Could you check a few things on this drawing? It's one solid part, dimensions in mm from its lowest x, y, z. A direction names the side the tool comes from. Coordinates: 2 decimals unless noted, no trailing zeros. Loops run counter-clockwise (first coordinate to the right, second up) from the corner with the lowest first, then second, coordinate; pieces in that order, holes last. Notation, with made-up numbers: (40, 77.5) -> (52, 77.5) arc R12 cw to (52, 98.5) -> close; hole circle Ø10 at (88, -15.5). An arc over 180 degrees is marked (long way). One line per question, with ' | ' between items. Start each with the question number.
(1) If we mould it in two halves opening along Z, with no side actions, what happens to the marked faces 1, 2 and 3? For each: pulls with the +Z half, pulls with the -Z half, needs draft (parallel to the pull), parting line crosses it, or undercut.
(2) I'm going to push flat-ended pins straight in: pin 1 Ø3 at (x, y) = (2.5, 4) entering from -Z; pin 2 Ø3 at (x, z) = (7.5, 1.5) entering from +Y; pin 3 Ø4 at (x, y) = (7, 6) entering from -Z; pin 4 Ø1 at (x, y) = (3.5, 3.5) entering from +Z. Where does each tip first touch, or does it pass through?
(3) Suppose I cut it at C-C (y = 1). Please give me the cut outline in (x, z), plus the area to 3 significant figures.
(4) Suppose I cut it at A-A (z = 7.5). Please give me the cut outline in (x, y) (1 decimal).
(5) Suppose I cut it at B-B (x = 6.25). Please give me the cut outline in (y, z) (1 decimal).
(6) Which directions (+Z, -Z, +X, -X, +Y, -Y) give clear straight access to the entire face, cutting with the end or side of a thin tool? Please do the marked faces 4 and 5.
(7) Suppose I cut it at D-D (x = 3.25). Please give me the cut outline in (y, z) (1 decimal), plus the area to 3 significant figures.
(8) If I drill on line 1 along Z through (x, y) = (5.5, 3.25) (1 decimal); line 2 along Y through (x, z) = (10.75, 6); line 3 along X through (y, z) = (5.5, 7.25) (1 decimal), over which ranges is the centre line in solid material (lowest first)?
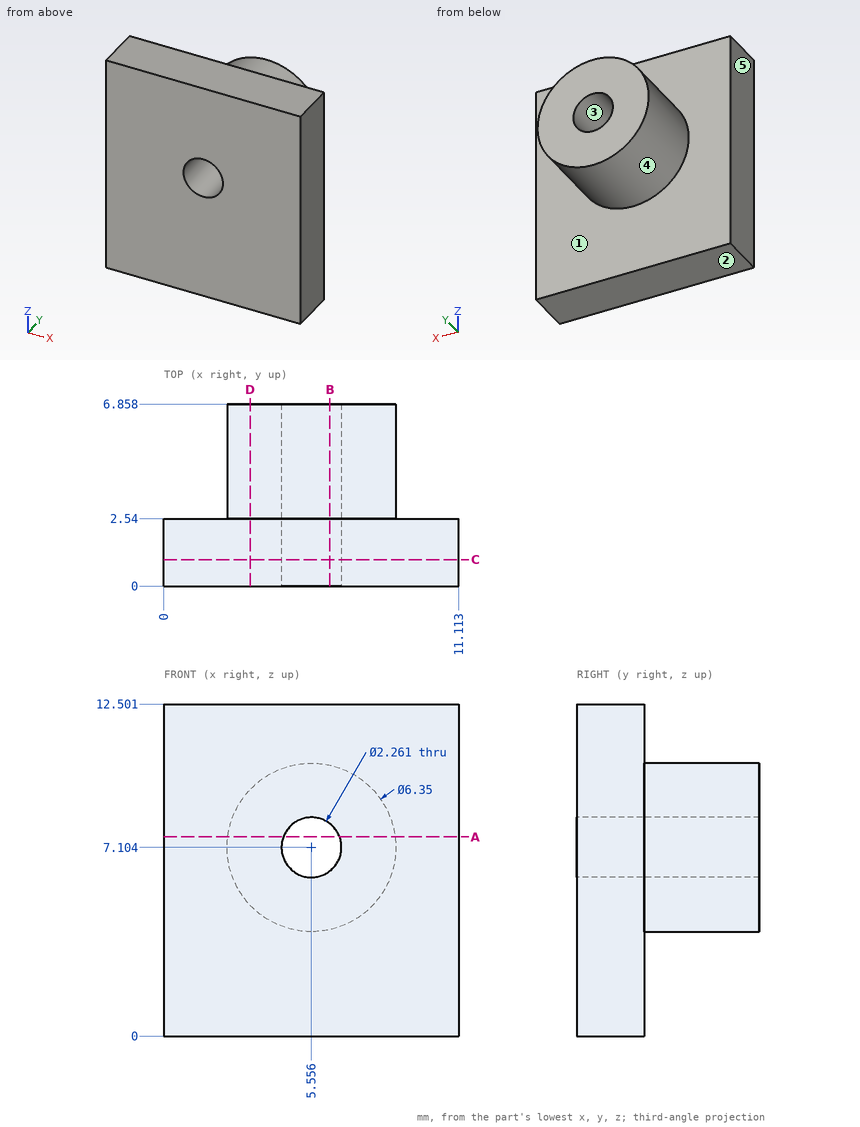
Checks:
1) face 1: needs draft | face 2: pulls with the -Z half | face 3: undercut
2) pin 1: stops at z = 0 | pin 2: stops at y = 2.54 | pin 3: stops at z = 3.93 | pin 4: stops at z = 9.87
3) outline: (0, 0) -> (11.11, 0) -> (11.11, 12.5) -> (0, 12.5) -> close; hole circle Ø2.26 at (5.56, 7.1) | area: 135 mm^2
4) outline: (0, 0) -> (4.5, 0) -> (4.5, 6.9) -> (2.4, 6.9) -> (2.4, 2.5) -> (0, 2.5) -> close; (6.6, 0) -> (11.1, 0) -> (11.1, 2.5) -> (8.7, 2.5) -> (8.7, 6.9) -> (6.6, 6.9) -> close
5) outline: (0, 0) -> (2.5, 0) -> (2.5, 4) -> (6.9, 4) -> (6.9, 6.2) -> (0, 6.2) -> close; (0, 8) -> (6.9, 8) -> (6.9, 10.2) -> (2.5, 10.2) -> (2.5, 12.5) -> (0, 12.5) -> close
6) face 4: +Y | face 5: +Z, -Z, -X, +Y, -Y
7) outline: (0, 0) -> (2.5, 0) -> (2.5, 4.9) -> (6.9, 4.9) -> (6.9, 9.3) -> (2.5, 9.3) -> (2.5, 12.5) -> (0, 12.5) -> close | area: 50.6 mm^2
8) line 1: z = 3.9 to 6, 8.2 to 10.3 | line 2: y = 0 to 2.54 | line 3: x = 2.4 to 4.4, 6.7 to 8.7
